Verification items for this drawing (mm, ordinates from the low corner). Give positions to 0.01 mm unless a question says otherwise; leave off trailing zeros. Loops run counter-clockwise (first coordinate to the right, second up) from the corner with the lowest first, then second, coordinate; pieces in that order, holes last. Notation, with made-up numbers: (85.25, 31.5) -> (103.25, 31.5) arc R14 ccw to (103.25, 35.5) -> close; hole circle Ø4 at (-35.75, -34.75). An arc over 180 degrees is marked (long way). Write each question's results on one line, items separated by ' | '. Start each with the question number.
Item 1: Mould release check, pull along X, two halves, no side actions. Record for the marked faces 1, 2 and 3: pulls with the +X half, pulls with the -X half, needs draft (parallel to the pull), parting line crosses it, or undercut.
Item 2: Cross-section at A-A on z = 10.5. Enter the section's corners in (x, y), then the cut area to 3 significant figures.
Item 3: Scan lines: line 1 along Y through (x, z) = (4, 10); line 2 along X through (y, z) = (4.5, 11.5); line 3 along X through (y, z) = (3.5, 2). Record each from-to range of solid material in increasing order.
Item 4: Gauge pin test, flat ends, axial feed: pin 1 Ø3 at (x, z) = (1.5, 3.5) entering from +Y; pin 2 Ø3 at (x, z) = (1, 5) entering from +Y; pin 3 Ø1.5 at (y, z) = (5.5, 8) entering from +X. Record the tip position at first contact, or that the pin passes through.
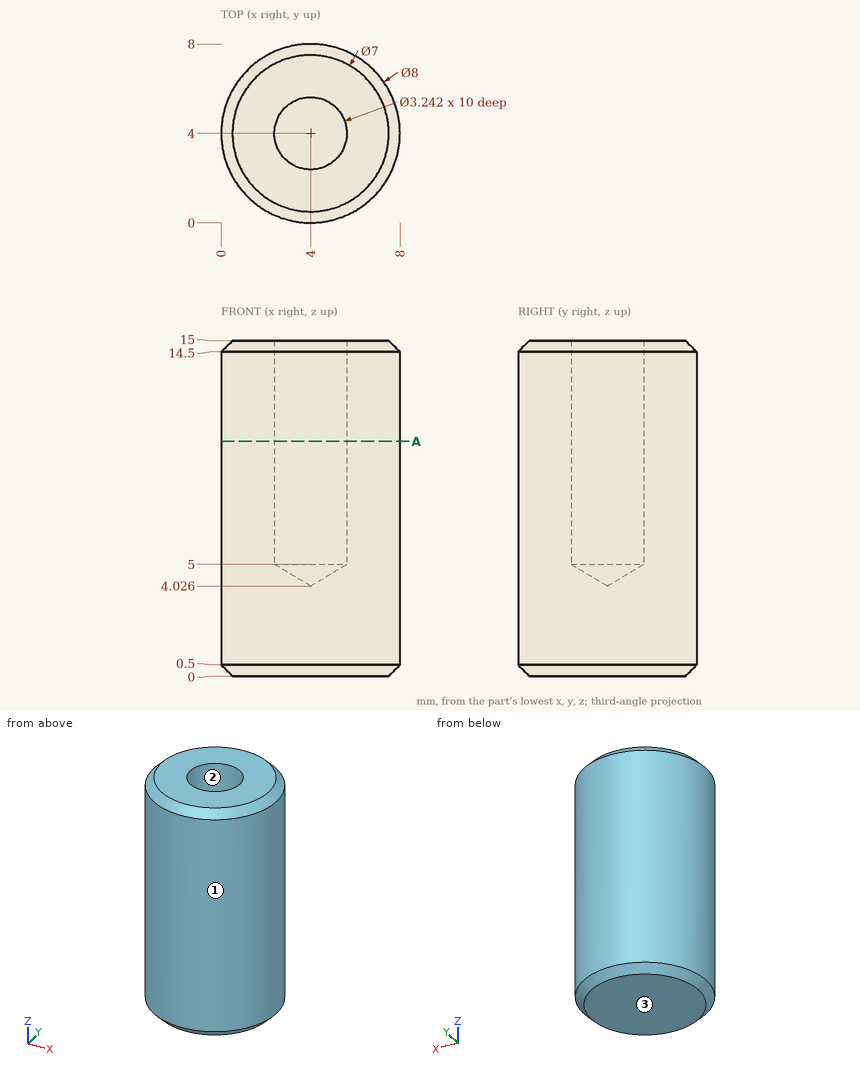
Answer sheet:
1) face 1: parting line crosses it | face 2: undercut | face 3: needs draft
2) outline: circle Ø8 at (4, 4); hole circle Ø3.24 at (4, 4) | area: 42.0 mm²
3) line 1: y = 0 to 2.38, 5.62 to 8 | line 2: x = 0.03 to 2.46, 5.54 to 7.97 | line 3: x = 0.03 to 7.97
4) pin 1: stops at y = 7.87 | pin 2: stops at y = 7.71 | pin 3: stops at x = 7.93
